Geometry: final body of the model. Coordinates: model frame, mm. A direction names the side the tool comes from. Round coordinates to 2 decimals unless told otherwise and drop trailing zeros. Write each loop counter-clockwise with the first axis right and the second up, starting at its lowest first coordinate (ties: lowest second). Pieces come first, ordered by that corner, then holes. Notation, with made-up numbers: (43, -33.75) - (60, -33.75) arc R10 cw to (60, -18.75) - close; hole circle Ø4 at (9, -9). An arc over 180 degrees is marked (long way). Write each question's results on one line, items separated by ' | '.
Solid Edge part; units mm, degrees
sketch "Sketch1" plane through (0, 0, 0) normal (0, 0, 1) x (1, 0, 0)
  line L0 (-108.956, -41.135) -> (108.956, -41.135)
  line L1 (108.956, -41.135) -> (108.956, 41.135)
  line L2 (108.956, 41.135) -> (-108.956, 41.135)
  line L3 (-108.956, 41.135) -> (-108.956, -41.135)
extrude "Protrusion1" add sketch "Sketch1" against normal blind 22
sketch "Sketch2" plane through (0, 0, 0) normal (0, 0, 1) x (0, 1, 0)
  line L0 (-41.135, -73.044) -> (-13.235, -73.044)
  line L1 (-13.235, -73.044) -> (41.135, -108.956)
  line L2 (41.135, -108.956) -> (-41.135, -108.956)
  line L3 (-41.135, -108.956) -> (-41.135, -73.044)
extrude "ExtrudedCutout_1" cut sketch "Sketch2" against normal blind 22
sketch "Sketch3" plane through (0, 0, 0) normal (0, 0, 1) x (1, 0, 0)
  line L0 (-108.956, 8.865) -> (108.956, 41.135)
  line L1 (108.956, 41.135) -> (-108.956, 41.135)
  line L2 (-108.956, 41.135) -> (-108.956, 8.865)
extrude "ExtrudedCutout_2" cut sketch "Sketch3" against normal blind 22
sketch "Sketch4" plane through (0, 0, 0) normal (0, 0, 1) x (1, 0, 0)
  circle A0 centre (-68.956, -21.135) radius 8
  circle A1 centre (31.044, -21.135) radius 8
extrude "ExtrudedCutout_3" cut sketch "Sketch4" against normal blind 22
Q1. Mould query, pull axis X, two halves, no side actions, for faces 3 (the flat face through (-2, -9, 0)), 4 (the cylindrical face through (38.434, -24.199, -10.846)), 5 (the cylindrical face through (-76.95, -20.78, -10.85)), 6 (the flat face through (-108.956, -16, -11)). Classes: pulls with the +X half, pulls with the -X half, needs draft (parallel to the pull), parting line crosses it, or undercut.
Answer block:
face 3: needs draft | face 4: undercut | face 5: undercut | face 6: pulls with the -X half
Q2. Section query B-B, the plane y = -24. Return loops of the section in (x, z).
Answer block:
outline: (-108.96, -22) - (-76.43, -22) - (-76.43, 0) - (-108.96, 0) - close; (-61.49, -22) - (23.57, -22) - (23.57, 0) - (-61.49, 0) - close; (38.51, -22) - (73.04, -22) - (73.04, 0) - (38.51, 0) - close
Q3. Ray query, line 1 along X through (y, z) = (-20.5, -5.75); line 2 along X through (y, z) = (-27.5, -14.5); line 3 along Y through (x, z) = (-75, -16.25) (3 decimals). Return the intervals inside material, ascending.
Answer block:
line 1: -108.96 to -76.93, -60.98 to 23.07, 39.02 to 73.04 | line 2: -108.96 to -73.8, -64.11 to 26.2, 35.89 to 73.04 | line 3: -41.135 to -26.376, -15.894 to 13.893
Q4. Section query A-A, the plane x = 26.5. Return loops of the section in (y, z) (3 decimals), plus the area to 3 significant figures.
Answer block:
outline: (-41.135, -22) - (-27.719, -22) - (-27.719, 0) - (-41.135, 0) - close; (-14.551, -22) - (28.924, -22) - (28.924, 0) - (-14.551, 0) - close | area: 1,250 mm2
Q5. Section query C-C, the plane z = -7. Return loops of the section in (x, y) (3 decimals).
Answer block:
outline: (-108.956, -41.135) - (73.044, -41.135) - (73.044, -13.235) - (108.956, 41.135) - (-108.956, 8.865) - close; hole circle Ø16 at (-68.956, -21.135); hole circle Ø16 at (31.044, -21.135)
Q6. Section query D-D, the plane x = 49.5. Return loops of the section in (y, z) (3 decimals), plus the area to 3 significant figures.
Answer block:
outline: (-41.135, -22) - (32.33, -22) - (32.33, 0) - (-41.135, 0) - close | area: 1,620 mm2
Q7. Access query for faces 1 (the flat face through (73.044, -27, -11)), 2 (the flat face through (-19, -41.135, -11)). Directions: +Z, -Z, +X, -X, +Y, -Y. A direction counts if a zero-diameter tool reaches every point of the face in a straight line with its end or side. Return the directions, or none.
Answer block:
face 1: +Z, -Z, +X, -Y | face 2: +Z, -Z, +X, -X, -Y
Q8. Pin query (flat end, axial travel): pin 1 (11 mm diameter, centred on y = -23, z = -10, fed in from +X); pin 2 (2 mm diameter, centred on y = 23.5, z = -13.5, fed in from +X); pin 3 (1 mm diameter, centred on y = -9, z = -11.5, fed in from +X). Return the tip coordinate at first contact, or that it passes through.
Answer block:
pin 1: x = 73.04 | pin 2: x = 97.97 | pin 3: x = 76.17
